The listing builds one solid part. Answer for the finished solid, in the listing's coordinates (mm). A direction names the side the tool comes from. Coordinates: 2 decimals unless noted, no trailing zeros. Write each loop counter-clockwise with the first axis right and the second up, starting at its lowest first coordinate (ties: lowest second). Pieces come first, ordered by that corner, then holes. Notation, with made-up numbers: M -20,-29 L 31,-29 A23 cw 31,-5 Z; hole C -21.5,66.5 d11. An arc over 180 degrees is marked long. Answer as CSV lines item,"result".
```python
from build123d import *

# Parameters (mm, degrees)
BOSS_EXTRUDE1_DEPTH = 20
SKETCH2_R           = 7.5
BOSS_EXTRUDE2_DEPTH = 5
SKETCH3_R           = 6.829132763
SKETCH3_R_2         = 6
BOSS_EXTRUDE3_DEPTH = 5


with BuildPart() as part:
    # Sketch1 → Boss-Extrude1 (new body)
    with BuildSketch(Plane(origin=(0, 0, 0), x_dir=(1, 0, 0), z_dir=(0, 1, 0))):
        with BuildLine():
            Line((-31.046293844, -29.276824699), (-60.108766173, -18.587025627))
            ThreePointArc((-60.108766173, -18.587025627), (-72.82850904, -3.124641863), (-65.560050374, 15.531367327))
            Line((-65.560050374, 15.531367327), (-41.175993118, 34.823361534))
            ThreePointArc((-41.175993118, 34.823361534), (-30.799217935, 39.089909616), (-19.738248933, 37.20952123))
            Line((-19.738248933, 37.20952123), (10.820861573, 22.53683551))
            ThreePointArc((10.820861573, 22.53683551), (24.755892372, -3.485081474), (4.178228718, -24.648375297))
            Line((4.178228718, -24.648375297), (-25.922904595, -29.750919304))
            ThreePointArc((-25.922904595, -29.750919304), (-28.515613019, -29.84902824), (-31.046293844, -29.276824699))
        make_face()
    extrude(amount=BOSS_EXTRUDE1_DEPTH)

    # Sketch2 → Boss-Extrude2 (add)
    with BuildSketch(Plane(origin=(0, 20, 0), x_dir=(1, 0, 0), z_dir=(0, 1, 0))):
        with Locations((-53.129573655, 0)):
            Circle(SKETCH2_R)
    extrude(amount=BOSS_EXTRUDE2_DEPTH)

    # Sketch3 → Boss-Extrude3 (add)
    with BuildSketch(Plane(origin=(0, 25, 0), x_dir=(1, 0, 0), z_dir=(0, 1, 0))):
        with Locations((-53.129573655, 0)):
            Circle(SKETCH3_R)
        with Locations((-53.129573655, 0)):
            Circle(SKETCH3_R_2, mode=Mode.SUBTRACT)
    extrude(amount=BOSS_EXTRUDE3_DEPTH)


solid = part.part
```
Q1. Find section A-A (z = 0). Give the vertices of the cut face in (x, y).
Output:
outline,"M -73.08,0 L 25,0 L 25,20 L -45.63,20 L -45.63,25 L -46.3,25 L -46.3,30 L -47.13,30 L -47.13,25 L -59.13,25 L -59.13,30 L -59.96,30 L -59.96,25 L -60.63,25 L -60.63,20 L -73.08,20 Z"
Q2. Flat-ended cylindrical pins translate along their axes: pin 1 Ø1.5 at (x, z) = (-38, 12) entering from +Y; pin 2 Ø12 at (y, z) = (16.5, 9) entering from -X; pin 3 Ø10 at (y, z) = (17.5, 20) entering from +X; pin 4 Ø5 at (y, z) = (24.5, 17) entering from -X. Find the tip coordinate at first contact, or state that the pin passes through.
Output:
pin 1,"y = 20"
pin 2,"x = -72.85"
pin 3,"x = 20"
pin 4,"through"
Q3. Find section B-B (y = 18.75). Give the vertices of the cut face in (x, z), and give its area (3 significant figures).
Output:
outline,"M -65.56,-15.53 L -41.18,-34.82 A20.35 ccw -19.74,-37.21 L 10.82,-22.54 A25 ccw 4.18,24.65 L -25.92,29.75 A10 ccw -31.05,29.28 L -60.11,18.59 A19.8 ccw Z"
area,"4,880 mm2"
Q4. Straight lines are drawn through the part: line 1 (X direction, y = 28.1, z = 0); line 2 (Y direction, x = -46.5, z = -26.5); line 3 (Z direction, x = -26, y = 9.75). For each, find the intervals that lie inside material, in ascending order.
Output:
line 1,"-59.96 to -59.13, -47.13 to -46.3"
line 2,"0 to 20"
line 3,"-39.05 to 29.76"
Q5. Find section D-D (x = 1.5). Give the vertices of the cut face in (y, z).
Output:
outline,"M 0,-27.01 L 20,-27.01 L 20,25.1 L 0,25.1 Z"
Q6. For faces 4 (the cylindrical face through (-46.616, 27.465, -2.051)), 5 (the cylindrical face through (-30.96, 9.86, -39.07)), determine the directions among +Z, -Z, +X, -X, +Y, -Y from which every point of the face is accessible in a straight line to the end or side of a thin tool.
Output:
face 4,"+Y"
face 5,"-Z, +Y, -Y"
Q7. The mould has two halves that part along X. Classify faces 1 (the flat face through (-49, 30, 5)), 2 (the flat face through (-53.54, 9.86, -25.04)), 3 (the cylindrical face through (-59.124, 27.465, -0.264)): pulls with the +X half, pulls with the -X half, needs draft (parallel to the pull), parting line crosses it, or undercut.
Output:
face 1,"needs draft"
face 2,"pulls with the -X half"
face 3,"undercut"
Q8. Find section C-C (y = 26.25). Give the vertices of the cut face in (x, z), and give its area (3 significant figures).
Output:
outline,"C -53.13,0 d13.66; hole C -53.13,0 d12"
area,"33.4 mm2"
